from build123d import *

# Parameters (mm, degrees)
SKETCH1_W           = 40
SKETCH1_H           = 80
SKETCH1_H_2         = 60
BOSS_EXTRUDE1_DEPTH = 2
SKETCH2_R           = 3
CUT_EXTRUDE1_DEPTH  = 5
CHAMFER1_SIZE       = 3


with BuildPart() as part:
    # Sketch1 → Boss-Extrude1 (new body, symmetric)
    with BuildSketch(Plane.XY):
        Rectangle(SKETCH1_W, SKETCH1_H)
        Polygon((20, -20), (20, -40), (60, -20), align=None)
        with Locations((40, 10)):
            Rectangle(SKETCH1_W, SKETCH1_H_2)
    extrude(amount=BOSS_EXTRUDE1_DEPTH, both=True)

    # Sketch2 → Cut-Extrude1 (cut, through all)
    with BuildSketch(Plane.XY.offset(2)):
        with Locations((50, 30)):
            Circle(SKETCH2_R)
        with Locations((30, 30)):
            Circle(SKETCH2_R)
        with Locations((50, -10)):
            Circle(SKETCH2_R)
        with Locations((30, -10)):
            Circle(SKETCH2_R)
        with Locations((-10, 30)):
            Circle(SKETCH2_R)
        with Locations((10, 30)):
            Circle(SKETCH2_R)
        with Locations((-10, 0)):
            Circle(SKETCH2_R)
        with Locations((10, 0)):
            Circle(SKETCH2_R)
        with Locations((-10, -30)):
            Circle(SKETCH2_R)
        with Locations((10, -30)):
            Circle(SKETCH2_R)
    extrude(amount=-CUT_EXTRUDE1_DEPTH, mode=Mode.SUBTRACT)

    # Chamfer1
    chamfer1_edges = [part.edges().sort_by_distance(p)[0] for p in [
        (7, 30, 2),
        (-13, 0, 2),
        (7, 0, 2),
        (-13, -30, 2),
        (27, 30, 2),
        (47, -10, 2),
        (27, -10, 2),
        (-13, 30, 2),
        (7, -30, 2),
        (47, 30, 2),
    ]]
    chamfer(chamfer1_edges, length=CHAMFER1_SIZE)


solid = part.part
The model under review builds one solid part; all positions refer to its coordinate system, in mm. Round coordinates to 2 decimals unless told otherwise and drop trailing zeros. Write each loop counter-clockwise with the first axis right and the second up, starting at its lowest first coordinate (ties: lowest second). Pieces come first, ordered by that corner, then holes. Notation, with made-up numbers: (13.25, 78.5) - (52.25, 78.5) arc R27 ccw to (52.25, 116.5) - close; hole circle Ø9 at (30, -29). An arc over 180 degrees is marked (long way). One line per item, written item: value. Start each with the question number.
1. Consider section A-A on x = 50. Write out the cut boundary in (y, z), and give its area (3 significant figures).
2. To check wall thickness, follow L1, parallel to Y at x = -10, z = -1.8; L2, parallel to Y at x = 30, z = -1.55; L3, parallel to X at y = 2, z = -1.65. State the ranges of each line that lie inside material, in increasing order. Write a range as from..to.
3. Consider section B-B on z = 1. State how many separate pieces and enclosed holes the cut face has, and give its area (3 significant figures).
4. Consider section D-D on y = 30. Write out the cut boundary in (x, z), and give its area (3 significant figures).
5. Consider section C-C on y = -30. Write out the cut boundary in (x, z), and give its area (3 significant figures).
6. Clearance check with flat-ended pins moving along their axes: P1, Ø7, axis at x = 10, y = 0, coming from the +Z side; P2, Ø5, axis at x = 50, y = 30, coming from the +Z side; P3, Ø9.5, axis at x = 10, y = 30, coming from the +Z side; P4, Ø8, axis at x = -10, y = 0, coming from the +Z side. State where each tip first meets the part, or that it passes through.
7. The part is to be moulded in two halves that separate along X. For faces 1 (the face through (-12.4, -31.8, -1.5)), 2 (the face through (-20, -1, 0)), 3 (the face through (0, -40, 0)), say which applies: released by +X, released by -X, zero draft, split by the parting line, or undercut.
Checks:
1. outline: (-25, -2) - (-13, -2) - (-13, -1) - (-16, 2) - (-25, 2) - close; (-7, -2) - (27, -2) - (27, -1) - (24, 2) - (-4, 2) - (-7, -1) - close; (33, -2) - (40, -2) - (40, 2) - (36, 2) - (33, -1) - close
1. area: 194 mm^2
2. L1: y = -40..-33, -27..-3, 3..27, 33..40
2. L2: y = -35..-13, -7..27, 33..40
2. L3: x = -20..-12.24, -7.76..7.76, 12.24..60
3. separate pieces: 1
3. enclosed holes: 10
3. area: 5,210 mm^2
4. outline: (-20, -2) - (-13, -2) - (-13, -1) - (-16, 2) - (-20, 2) - close; (-7, -2) - (7, -2) - (7, -1) - (4, 2) - (-4, 2) - (-7, -1) - close; (13, -2) - (27, -2) - (27, -1) - (24, 2) - (16, 2) - (13, -1) - close; (33, -2) - (47, -2) - (47, -1) - (44, 2) - (36, 2) - (33, -1) - close; (53, -2) - (60, -2) - (60, 2) - (56, 2) - (53, -1) - close
4. area: 188 mm^2
5. outline: (-20, -2) - (-13, -2) - (-13, -1) - (-16, 2) - (-20, 2) - close; (-7, -2) - (7, -2) - (7, -1) - (4, 2) - (-4, 2) - (-7, -1) - close; (13, -2) - (40, -2) - (40, 2) - (16, 2) - (13, -1) - close
5. area: 174 mm^2
6. P1: stops at z = -0.5
6. P2: passes through
6. P3: stops at z = 0.75
6. P4: stops at z = 0
7. face 1: undercut
7. face 2: released by -X
7. face 3: zero draft
